Read the model definition and answer for the solid it produces. Units are mm, in the model's axes. A direction names the side the tool comes from. Give positions to 0.01 mm unless a question says otherwise; leave off trailing zeros. Order: outer loops, then holes, each group sorted by start corner. A loop starts at its lowest first (then second) coordinate and runs counter-clockwise, first axis right, second up.
Item 1: Which of the six approach directions +Z, -Z, +X, -X, +Y, -Y give full straight-line access (tool end or side, diameter ignored) to faces 1 (the face through (-178.5, -3, 15)), 2 (the face through (145.96, -3, 16))?
Item 2: Given pin 1 Ø2 at (x, y) = (-97, 170.5) entering from +Z, flat-ended and moving along its own axis, determine where the tip first touches the part or whether it passes through.
Item 3: A cutting plane is placed at C-C (y = 182). Write down the section's boundary in (x, z), plus the area to 3 significant figures.
Item 4: A cutting plane is placed at B-B (x = 85.5). Write down the section's boundary in (y, z), plus the area to 3 significant figures.
Item 5: Find the intervals of material crossed by line 1 along X through (y, z) = (103, 11.25); line 2 along Y through (x, z) = (2, 20.5); line 3 along Z through (x, y) = (91.5, -143.5), in increasing order.
Item 6: A cutting plane is placed at A-A (z = 12.5). Write down the section's boundary in (x, y), plus the area to 3 significant figures.
Item 7: The mould has two halves that part along Y. Classify faces 3 (the face through (-2, 207.46, 16)), 4 (the face through (-2, -240, 15)), 5 (the face through (-2, 3, 0)), 6 (the face through (-2, 240, 15)): +Y half, -Y half, draft (parallel to the pull), parting line (faces both ways), or undercut.
from build123d import *

# Parameters (mm, degrees)
F0_W     = 357
F0_H     = 480
F1_DEPTH = 30
F2_T     = -2.54
F3_DEPTH = 30
F4_DEPTH = 30
F5_DEPTH = 30
F6_DEPTH = 30


with BuildPart() as f1:
    # F0 (on Top) → F1 (new body)
    with BuildSketch(Plane.XY):
        Rectangle(F0_W, F0_H)
    extrude(amount=F1_DEPTH)

    # F2
    f2_openings = [f1.faces().sort_by_distance(p)[0] for p in [
        (0, 0, 30),
    ]]
    offset(amount=F2_T, openings=f2_openings)

    # F3 (add): a face of the model
    f3_faces = [f1.faces().sort_by_distance(p)[0] for p in [
        (0, 237.46, 16.27),
    ]]
    extrude(f3_faces, amount=F3_DEPTH)

    # F4 (add): a face of the model
    f4_faces = [f1.faces().sort_by_distance(p)[0] for p in [
        (175.96, -15, 16.27),
    ]]
    extrude(f4_faces, amount=F4_DEPTH)

    # F5 (add): a face of the model
    f5_faces = [f1.faces().sort_by_distance(p)[0] for p in [
        (-175.96, -15, 16.27),
    ]]
    extrude(f5_faces, amount=F5_DEPTH)

    # F6 (add): a face of the model
    f6_faces = [f1.faces().sort_by_distance(p)[0] for p in [
        (0, -237.46, 16.27),
    ]]
    extrude(f6_faces, amount=F6_DEPTH)


solid = f1.part
Response values:
1. face 1: +Z, -Z, -X, +Y, -Y
1. face 2: +Z
2. pin 1: stops at z = 2.54
3. outline: (-178.5, 0) - (178.5, 0) - (178.5, 30) - (145.96, 30) - (145.96, 2.54) - (-145.96, 2.54) - (-145.96, 30) - (-178.5, 30) - close
3. area: 2,690 mm2
4. outline: (-240, 0) - (240, 0) - (240, 30) - (207.46, 30) - (207.46, 2.54) - (-207.46, 2.54) - (-207.46, 30) - (-240, 30) - close
4. area: 3,010 mm2
5. line 1: x = -178.5 to -145.96, 145.96 to 178.5
5. line 2: y = -240 to -207.46, 207.46 to 240
5. line 3: z = 0 to 2.54
6. outline: (-178.5, -240) - (178.5, -240) - (178.5, 240) - (-178.5, 240) - close; hole (-145.96, -207.46) - (145.96, -207.46) - (145.96, 207.46) - (-145.96, 207.46) - close
6. area: 50,200 mm2
7. face 3: undercut
7. face 4: -Y half
7. face 5: draft
7. face 6: +Y half
